Part model, mm, in its own coordinate system. A direction names the side the tool comes from. Coordinates: 2 decimals unless noted, no trailing zeros. Write each loop counter-clockwise with the first axis right and the second up, starting at its lowest first coordinate (ties: lowest second). Pieces come first, ordered by that corner, then holes. Notation, with made-up numbers: M 46,-1 L 60,-1 A25 ccw 60,15 Z; hole C -20,35 d9. An arc over 180 degrees is marked long. Use a Markdown table: item, result. Add a question column.
Q1. Pin check, flat tips, straight feed: pin 1 Ø10 at (y, z) = (33.5, 13.5) entering from -X; pin 2 Ø6 at (x, z) = (10.5, 13) entering from +Y; pin 3 Ø3 at (y, z) = (20.5, 5.5) entering from +X. Stop position of each tip, or through.
Q2. Slice it at B-B on y = 3. Write the cut outline in (x, z).
Q3. Slice it at D-D on z = -10. Write the cut outline in (x, y), then the cut area to 3 significant figures.
Q4. Slice it at C-C on z = 2.5. Write the cut outline in (x, y) (3 decimals).
Q5. Slice it at A-A on x = 12. Write the cut outline in (y, z).
Q6. Tool access for faces 1 (the flat face through (10, 0, 0)), 2 (the flat face through (10, 30, 0)): list every direction of +Z, -Z, +X, -X, +Y, -Y with a clear straight run to the whole face (end or side of a thin tool).
Q7. Wall check: L1, parallel to Y at x = 17, z = 4; L2, parallel to Y at x = 17.5, z = -12; L3, parallel to X at y = 11, z = 12.5 (1 decimal). Give the ranges that are in metal, low to high. Write a range as from..to.
Autodesk Inventor part; units mm, degrees
ref_plane "YZ Plane" through (0, 0, 0) normal (1, 0, 0) x (0, 1, 0)
ref_plane "XZ Plane" through (0, 0, 0) normal (0, 1, 0) x (-1, 0, 0)
ref_plane "XY Plane" through (0, 0, 0) normal (0, 0, 1) x (1, 0, 0)
sketch "草圖1" plane through (0, 0, 0) normal (0, 1, 0) x (-1, 0, 0)
  circle A0 centre (0, 0) radius 20
  line L0 (0, -20) -> (-40, -20)
  line L1 (-40, -20) -> (-40, 20)
  line L2 (-40, 20) -> (0, 20)
  line L3 (0, 20) -> (0, -20)
  point P0 (0, 20)
  dimension "d0" = 40
  dimension "d1" = 40
extrude "擠出1" add sketch "草圖1" along normal blind 40
sketch "草圖2" plane through (0, 40, 0) normal (0, 1, 0) x (1, 0, 0)
  line L0 (0, 20) -> (40, 20)
  line L1 (40, 20) -> (40, -20)
  line L2 (40, -20) -> (0, -20)
  arc A0 (0, 20) -> (0, -20) centre (0, 0) ccw
  line L3 (0, -20) -> (40, -20)
  line L4 (40, -20) -> (30, 20)
  dimension "d4" = 10
extrude "擠出2" cut sketch "草圖2" against normal through all contours L0 L1 L4
sketch "草圖3" plane through (0, 40, 0) normal (0, 1, 0) x (1, 0, 0)
  line L0 (30, 20) -> (0, 20)
  line L1 (20, 20) -> (10, -20)
  line L2 (0, -20) -> (40, -20)
  line L3 (30, 20) -> (40, -20)
  line L4 (40, -20) -> (0, -20)
  arc A0 (0, 20) -> (0, -20) centre (0, 0) ccw
  line L5 (0, 20) -> (30, 20)
  dimension "d7" = 10
  dimension "d8" = 30
extrude "擠出3" cut sketch "草圖3" against normal blind 30 contours L3 L2 L1 L0
sketch "草圖4" plane through (0, 40, 0) normal (0, 1, 0) x (1, 0, 0)
  line L0 (20, 20) -> (10, -20)
  line L1 (10, -20) -> (0, -20)
  arc A0 (0, 20) -> (0, -20) centre (0, 0) ccw
  line L2 (0, 20) -> (20, 20)
  line L3 (20, 20) -> (0, 20)
  line L4 (9.6922, 20) -> (-0.3072, -19.9976)
  line L5 (0, -20) -> (40, -20)
  line L6 (10, -20) -> (20, 20)
  dimension "d11" = 10
extrude "擠出4" cut sketch "草圖4" against normal blind 10 contours L0 L1 A0 L4 L2
properties part number "6" material "鋼、碳鋼"
Recorded:
| question | item | result |
|---|---|---|
| 1 | pin 1 | x = -18.1 |
| 1 | pin 2 | y = 30 |
| 1 | pin 3 | x = 14 |
| 2 | outline | M 0,-20 L 30,-20 L 40,20 L 0,20 A20 ccw Z |
| 3 | outline | M -17.32,0 L 32.5,0 L 32.5,10 L 17.5,10 L 17.5,30 L 7.19,30 L 7.19,40 L -17.32,40 Z |
| 3 | area | 1,440 mm² |
| 4 | outline | M -19.843,0 L 35.625,0 L 35.625,10 L 14.375,10 L 14.375,30 L 4.067,30 L 4.067,40 L -19.843,40 Z |
| 5 | outline | M 0,-20 L 30,-20 L 30,12 L 10,12 L 10,20 L 0,20 Z |
| 6 | face 1 | +Z, -Z, +X, -X, -Y |
| 6 | face 2 | +Z, +X, +Y |
| 7 | L1 | 0..10 |
| 7 | L2 | 0..30 |
| 7 | L3 | -15.6..11.9 |
